```python
from build123d import *

# Parameters (mm, degrees)
ESQUISSE1_W        = 3
ESQUISSE1_H        = 8
BOSS_EXTRU_1_DEPTH = 3
CONG_1_R           = 20


with BuildPart() as part:
    # Esquisse1 → Boss.-Extru.1 (new body)
    with BuildSketch(Plane.XY):
        Polygon((-68.936542711, 42.155372437), (-9.179039763, 36.766416935), (0, 0), (-68.936542711, 12.155372437), align=None)
        with Locations((-70.436542711, 38.155372437)):
            Rectangle(ESQUISSE1_W, ESQUISSE1_H)
        with Locations((-70.436542711, 27.155372437)):
            Rectangle(ESQUISSE1_W, ESQUISSE1_H)
        with Locations((-70.436542711, 16.155372437)):
            Rectangle(ESQUISSE1_W, ESQUISSE1_H)
    extrude(amount=BOSS_EXTRU_1_DEPTH)

    # Congé1
    cong_1_edges = [part.edges().sort_by_distance(p)[0] for p in [
        (-9.179039763, 36.766416935, 1.5),
    ]]
    fillet(cong_1_edges, radius=CONG_1_R)


solid = part.part
```
CAD build for the part. Positions are in the model's coordinates, mm. A direction names the side the tool comes from. Give positions to 0.01 mm unless a question says otherwise; leave off trailing zeros. Order: outer loops, then holes, each group sorted by start corner. A loop starts at its lowest first (then second) coordinate and runs counter-clockwise, first axis right, second up. Notation, with made-up numbers: M 4.25,54 L 14.25,54 A34 ccw 14.25,90 Z; hole C 55,2 d4. An arc over 180 degrees is marked long. Put each result on its own line as item: value. Start each with the question number.
(1) Drill centre lines: line 1 along Y through (x, z) = (-41, 2.2); line 2 along Y through (x, z) = (-39, 2.3); line 3 along X through (y, z) = (14, 0.4). Where is each one in solid material? Low to high.
(2) Saw through at A-A, the plane z = 0.55. Write the cut outline in (x, y), then the cut area to 3 significant figures.
(3) Saw through at B-B, the plane y = 21. Write the cut outline in (x, z), then the cut area to 3 significant figures.
(4) Saw through at C-C, the plane x = -62. Write the cut outline in (y, z).
(5) Which spindle directions (+Z, -Z, +X, -X, +Y, -Y) get a long thin tool onto all of the face, cutting with end or side? Do faces 4 (the flat face through (-35, 21, 0)), 5 (the flat face through (-70, 23.155, 1)). Say none if no direction does.
(6) Mould opens along Y. For faces 1 (the flat face through (-2.91, 11.65, 1.48)), 2 (the flat face through (-68.937, 33, 1)), 3 (the flat face through (-70, 12.155, 1)) say: +Y half, -Y half, draft (parallel to the pull), parting line (faces both ways), or undercut.
(7) Flat gauge pins, fed straight in: pin 1 Ø1.5 at (x, z) = (-70, 1) entering from -Y; pin 2 Ø1.5 at (y, z) = (5, 1) entering from +X. Where does each tip first touch, or does it go through?
Check result:
1. line 1: y = 7.23 to 39.64
1. line 2: y = 6.88 to 39.46
1. line 3: x = -71.94 to -3.5
2. outline: M -71.94,12.16 L -68.94,12.16 L 0,0 L -5.73,22.97 A20 ccw -23.34,38.04 L -68.94,42.16 L -71.94,42.16 L -71.94,34.16 L -68.94,34.16 L -68.94,31.16 L -71.94,31.16 L -71.94,23.16 L -68.94,23.16 L -68.94,20.16 L -71.94,20.16 Z
2. area: 2,140 mm2
3. outline: M -68.94,0 L -5.24,0 L -5.24,3 L -68.94,3 Z
3. area: 191 mm2
4. outline: M 10.93,0 L 41.53,0 L 41.53,3 L 10.93,3 Z
5. face 4: -Z, +X, -X, +Y, -Y
5. face 5: +Z, -Z, -X
6. face 1: +Y half
6. face 2: undercut
6. face 3: -Y half
7. pin 1: stops at y = 12.16
7. pin 2: stops at x = -1.06
